Geometry: final body of the model. Coordinates: model frame, mm. A direction names the side the tool comes from. Round coordinates to 2 decimals unless told otherwise and drop trailing zeros. Loops run counter-clockwise (first coordinate to the right, second up) from the corner with the lowest first, then second, coordinate; pieces in that order, holes last. Notation, with made-up numbers: (50.25, 79) -> (97.25, 79) arc R15 cw to (97.25, 104) -> close; hole circle Ø4 at (60, -18.75). An arc over 180 degrees is marked (long way). Answer in a Markdown table with one row per item.
```python
from build123d import *

# Parameters (mm, degrees)
SKETCH1_W               = 90
SKETCH1_H               = 100
BOSS_EXTRUDE1_DEPTH     = 40
SKETCH3_W               = 25
SKETCH3_H               = 40
BOSS_EXTRUDE3_DEPTH     = 10
SKETCH5_W               = 15
SKETCH5_H               = 20
CUT_EXTRUDE1_DEPTH      = 10
SKETCH6_W               = 25
SKETCH6_H               = 10
BOSS_EXTRUDE4_DEPTH     = 10
SKETCH7_W               = 10
SKETCH7_H               = 30
CUT_EXTRUDE2_DEPTH      = 15
CUT_EXTRUDE3_DEPTH      = 108.861822617
CUT_EXTRUDE3_DEPTH_BACK = 108.861822617
SKETCH8_R               = 1.7
SKETCH9_R               = 1.7
CUT_EXTRUDE4_DEPTH      = 57


with BuildPart() as part:
    # Sketch1 → Boss-Extrude1 (new body)
    with BuildSketch(Plane(origin=(0, 0, 0), x_dir=(1, 0, 0), z_dir=(0, 1, 0))):
        with BuildLine():
            Line((-45.284100543, 33.309612736), (34.715899457, 33.309612736))
            ThreePointArc((34.715899457, 33.309612736), (45.322501175, 28.916214454), (49.715899457, 18.309612736))
            Line((49.715899457, 18.309612736), (49.715899457, -71.690387264))
            ThreePointArc((49.715899457, -71.690387264), (45.322501175, -82.296988982), (34.715899457, -86.690387264))
            Line((34.715899457, -86.690387264), (-45.284100543, -86.690387264))
            ThreePointArc((-45.284100543, -86.690387264), (-55.890702261, -82.296988982), (-60.284100543, -71.690387264))
            Line((-60.284100543, -71.690387264), (-60.284100543, 18.309612736))
            ThreePointArc((-60.284100543, 18.309612736), (-55.890702261, 28.916214454), (-45.284100543, 33.309612736))
        make_face()
        with Locations((-5.284100543, -26.690387264)):
            Rectangle(SKETCH1_W, SKETCH1_H, mode=Mode.SUBTRACT)
    extrude(amount=BOSS_EXTRUDE1_DEPTH)

    # Sketch3 → Boss-Extrude3 (add)
    with BuildSketch(Plane(origin=(0, 40, 0), x_dir=(1, 0, 0), z_dir=(0, 1, 0))):
        with Locations((-47.784100543, -26.690387264)):
            Rectangle(SKETCH3_W, SKETCH3_H)
    extrude(amount=-BOSS_EXTRUDE3_DEPTH)

    # Sketch5 → Cut-Extrude1 (cut)
    with BuildSketch(Plane(origin=(0, 40, 0), x_dir=(1, 0, 0), z_dir=(0, 1, 0))):
        with Locations((-42.784100543, -26.690387264)):
            Rectangle(SKETCH5_W, SKETCH5_H)
    extrude(amount=-CUT_EXTRUDE1_DEPTH, mode=Mode.SUBTRACT)

    # Sketch6 → Boss-Extrude4 (add)
    with BuildSketch(Plane(origin=(0, 40, 0), x_dir=(1, 0, 0), z_dir=(0, 1, 0))):
        with Locations((37.215899457, -46.690387264)):
            Rectangle(SKETCH6_W, SKETCH6_H)
        with Locations((37.215899457, -6.690387264)):
            Rectangle(SKETCH6_W, SKETCH6_H)
    extrude(amount=-BOSS_EXTRUDE4_DEPTH)

    # Sketch7 → Cut-Extrude2 (cut)
    with BuildSketch(Plane(origin=(0, 40, 0), x_dir=(1, 0, 0), z_dir=(0, 1, 0))):
        with Locations((-55.284100543, 8.309612736)):
            Rectangle(SKETCH7_W, SKETCH7_H)
        with Locations((-55.284100543, -61.690387264)):
            Rectangle(SKETCH7_W, SKETCH7_H)
        with Locations((44.715899457, -26.690387264)):
            Rectangle(SKETCH7_W, SKETCH7_H)
    extrude(amount=-CUT_EXTRUDE2_DEPTH, mode=Mode.SUBTRACT)

    # Sketch8 → Cut-Extrude3 (cut, two sides: drawn at the far end of the back side and taken through both)
    with BuildSketch(Plane.XY.offset(46.690387264).offset(-CUT_EXTRUDE3_DEPTH_BACK)):
        with Locations((-42.784100543, 35)):
            Circle(SKETCH8_R)
    extrude(amount=CUT_EXTRUDE3_DEPTH + CUT_EXTRUDE3_DEPTH_BACK, mode=Mode.SUBTRACT)

    # Sketch9 → Cut-Extrude4 (cut)
    with BuildSketch(Plane.XY.offset(51.690387264)):
        with Locations((32.215899457, 35)):
            Circle(SKETCH9_R)
    extrude(amount=-CUT_EXTRUDE4_DEPTH, mode=Mode.SUBTRACT)


solid = part.part
```
Item 1: Pin query (flat end, axial travel): pin 1 Ø3 at (x, z) = (32, 45) entering from -Y; pin 2 Ø8 at (x, z) = (-55, 64.5) entering from +Y. Return the tip coordinate at first contact, or that it passes through.
Answer:
| item | result |
|---|---|
| pin 1 | stops at y = 30 |
| pin 2 | stops at y = 25 |
Item 2: Cut plane B-B (z = 29.5). Output: boundary loops of the cut face in (x, y), then the cut area to 3 significant figures.
Answer:
| item | result |
|---|---|
| outline | (-60.28, 0) -> (-50.28, 0) -> (-50.28, 40) -> (-60.28, 40) -> close; (39.72, 0) -> (49.72, 0) -> (49.72, 25) -> (39.72, 25) -> close |
| area | 650 mm² |
Item 3: Draft query along X for faces 5 (the face through (30, 35, 1.69)), 6 (the face through (49.716, 20, 27)), 7 (the face through (33.786, 34.349, 46.76)). Return one class per face: pulls with the +X half, pulls with the -X half, needs draft (parallel to the pull), parting line crosses it, or undercut.
Answer:
| item | result |
|---|---|
| face 5 | needs draft |
| face 6 | pulls with the +X half |
| face 7 | undercut |
Item 4: Cut plane C-C (x = -27). Output: boundary loops of the cut face in (y, z), then the cut area to 3 significant figures.
Answer:
| item | result |
|---|---|
| outline | (0, -33.31) -> (40, -33.31) -> (40, -23.31) -> (0, -23.31) -> close; (0, 76.69) -> (40, 76.69) -> (40, 86.69) -> (0, 86.69) -> close |
| area | 800 mm² |
Item 5: Line query: probe 1 along Z at (x, y) = (13, 14.5); probe 2 along X at (y, z) = (19.5, -1); probe 3 along Y at (x, z) = (-42.5, -24). Output: solid intervals per line, ascending. Write a range as [from, to].
Answer:
| item | result |
|---|---|
| probe 1 | z = [-33.31, -23.31], [76.69, 86.69] |
| probe 2 | x = [-60.28, -50.28], [39.72, 49.72] |
| probe 3 | y = [0, 33.32], [36.68, 40] |
Item 6: Cut plane A-A (z = 50). Output: boundary loops of the cut face in (x, y), then the cut area to 3 significant figures.
Answer:
| item | result |
|---|---|
| outline | (-60.28, 0) -> (-50.28, 0) -> (-50.28, 25) -> (-60.28, 25) -> close; (24.72, 30) -> (39.72, 30) -> (39.72, 0) -> (49.72, 0) -> (49.72, 40) -> (24.72, 40) -> close; hole circle Ø3.4 at (32.22, 35) |
| area | 791 mm² |
Item 7: Reachability of faces 1 (the face through (-45, 35, 36.69)), 2 (the face through (39.716, 15, 27)), 3 (the face through (-55, 25, -9)), 4 (the face through (40, 34, 41.69)) from +Z, -Z, +X, -X, +Y, -Y: full face, straight path, thin tool, end or side. Return the list, or none.
Answer:
| item | result |
|---|---|
| face 1 | +X, +Y, -Y |
| face 2 | -Y |
| face 3 | -X, +Y |
| face 4 | +X, +Y |
Item 8: Cut plane D-D (x = -39.5). Output: boundary loops of the cut face in (y, z), then the cut area to 3 significant figures.
Answer:
| item | result |
|---|---|
| outline | (0, -33.31) -> (40, -33.31) -> (40, -23.31) -> (0, -23.31) -> close; (0, 76.69) -> (40, 76.69) -> (40, 86.69) -> (0, 86.69) -> close; (30, 6.69) -> (40, 6.69) -> (40, 16.69) -> (30, 16.69) -> close; (30, 36.69) -> (40, 36.69) -> (40, 46.69) -> (30, 46.69) -> close |
| area | 1,000 mm² |
